from build123d import *

# Parameters (mm, degrees)
EXTRUDE_1_DEPTH    = 6
HOLE_WIZARD_M3_1_D = 2.5
HOLE_WIZARD_M3_2_D = 2.5


with BuildPart() as part:
    # 草图1 → 凸台-拉伸1 (new body)
    with BuildSketch(Plane.XY):
        Polygon((0, 0), (0, -3), (10, -3), (10, 7), (7, 7), (7, 0), align=None)
    extrude(amount=EXTRUDE_1_DEPTH)

    # M3 螺纹孔1 (through all)
    with Locations(Plane(origin=(0, -3, 0), x_dir=(-1, 0, 0), z_dir=(0, -1, 0))):
        with Locations((-5, -3)):
            Hole(HOLE_WIZARD_M3_1_D / 2)

    # M3 螺纹孔2 (through all)
    with Locations(Plane(origin=(10, 0, 0), x_dir=(0, 0, -1), z_dir=(1, 0, 0))):
        with Locations((-3, 2)):
            Hole(HOLE_WIZARD_M3_2_D / 2)


solid = part.part
Verification items for the finished model (mm, model axes). A direction names the side the tool comes from. Round coordinates to 2 decimals unless told otherwise and drop trailing zeros. Loops run counter-clockwise (first coordinate to the right, second up) from the corner with the lowest first, then second, coordinate; pieces in that order, holes last. Notation, with made-up numbers: (74.5, 42.5) - (91.5, 42.5) arc R14 cw to (91.5, 58.5) - close; hole circle Ø2 at (10.5, 18.5). An arc over 180 degrees is marked (long way). Use a Markdown table: item, result. Add a question column.
1. Thickness scan on probe 1 along Y at (x, z) = (8.1, 3); probe 2 along X at (y, z) = (4, 5.3); probe 3 along Y at (x, z) = (1.5, 3.4). Record the ranges inside material, lowest first. Write a range as [from, to].
2. Section check A-A, the plane y = 2. Record the boundary of the cut face in (x, z), plus the area to 3 significant figures.
3. Section check D-D, the plane z = 0.6. Record the boundary of the cut face in (x, y), plus the area to 3 significant figures.
4. Release check for a two-part mould opening along Z. For faces 3 (the face through (6, -0.2, 6)), 4 (the face through (10, 1, 2)), 5 (the face through (4.079, -1.479, 2.155)) record: released by +Z, released by -Z, zero draft, split by the parting line, or undercut.
5. Section check B-B, the plane x = 5. Record the boundary of the cut face in (y, z), plus the area to 3 significant figures.
6. Section check C-C, the plane z = 3. Record the boundary of the cut face in (x, y), plus the area to 3 significant figures.
7. Access from +Z, -Z, +X, -X, +Y, -Y to the whole of each face (thin tool, end or side, straight path). Record for faces 1 (the face through (7, 4, 3)), 2 (the face through (9, 7, 3)).
8. Gauge pin test, flat ends, axial feed: pin 1 (3 mm diameter, centred on x = 5, z = 3, fed in from +Y); pin 2 (1.8 mm diameter, centred on y = 5, z = 2.5, fed in from -X). Record the tip position at first contact, or that the pin passes through.
Checks:
| question | item | result |
|---|---|---|
| 1 | probe 1 | y = [-3, 0.75], [3.25, 7] |
| 1 | probe 2 | x = [7, 10] |
| 1 | probe 3 | y = [-3, 0] |
| 2 | outline | (7, 0) - (10, 0) - (10, 1.75) - (7, 1.75) - close; (7, 4.25) - (10, 4.25) - (10, 6) - (7, 6) - close |
| 2 | area | 10.5 mm^2 |
| 3 | outline | (0, -3) - (10, -3) - (10, 7) - (7, 7) - (7, 0) - (0, 0) - close |
| 3 | area | 51.0 mm^2 |
| 4 | face 3 | released by +Z |
| 4 | face 4 | zero draft |
| 4 | face 5 | undercut |
| 5 | outline | (-3, 0) - (0, 0) - (0, 1.75) - (-3, 1.75) - close; (-3, 4.25) - (0, 4.25) - (0, 6) - (-3, 6) - close |
| 5 | area | 10.5 mm^2 |
| 6 | outline | (0, -3) - (3.75, -3) - (3.75, 0) - (0, 0) - close; (6.25, -3) - (10, -3) - (10, 0.75) - (7, 0.75) - (7, 0) - (6.25, 0) - close; (7, 3.25) - (10, 3.25) - (10, 7) - (7, 7) - close |
| 6 | area | 36.0 mm^2 |
| 7 | face 1 | +Z, -Z, -X, +Y |
| 7 | face 2 | +Z, -Z, +X, -X, +Y |
| 8 | pin 1 | stops at y = 0 |
| 8 | pin 2 | stops at x = 7 |
